Here's how the part is built. I have some questions about the finished solid (model axes, mm). A direction names the side the tool comes from. Coordinates: 2 decimals unless noted, no trailing zeros. Put each result on its own line as item: value.
```python
from build123d import *

# Parameters (mm, degrees)
SKETCH1_R           = 1.35
SKETCH1_R_2         = 1.3
BOSS_EXTRUDE1_DEPTH = 15.5
CUT_EXTRUDE1_DEPTH  = 6
FILLET1_R           = 3
CHAMFER1_SIZE       = 1.5
SKETCH3_W           = 7.93
SKETCH3_H           = 22
CUT_EXTRUDE2_DEPTH  = 8.3
SKETCH4_W           = 64.15
SKETCH4_H           = 2
CUT_EXTRUDE3_DEPTH  = 8.3


with BuildPart() as part:
    # Sketch1 → Boss-Extrude1 (new body)
    with BuildSketch(Plane.XY):
        with BuildLine():
            Line((-36.4, 19.96), (-36.4, 28))
            Line((-36.4, 28), (-39.5, 28))
            ThreePointArc((-39.5, 28), (-41.621320344, 27.121320344), (-42.5, 25))
            Line((-42.5, 25), (-42.5, -25))
            ThreePointArc((-42.5, -25), (-41.621320344, -27.121320344), (-39.5, -28))
            Line((-39.5, -28), (27.64, -28))
            Line((27.64, -28), (27.64, 8.8))
            Line((27.64, 8.8), (23.15, 8.8))
            Line((23.15, 8.8), (23.15, 28))
            Line((23.15, 28), (16.4, 28))
            Line((16.4, 28), (16.4, 21.51))
            Line((16.4, 21.51), (22.004438923, 21.51))
            Line((22.004438923, 21.51), (22.004438923, 15.51))
            Line((22.004438923, 15.51), (16.004438923, 15.51))
            Line((16.004438923, 15.51), (16.004438923, 19.96))
            Line((16.004438923, 19.96), (-36.4, 19.96))
        make_face()
        with Locations((-39, -24.5)):
            Circle(SKETCH1_R, mode=Mode.SUBTRACT)
        with Locations((19, -24.5)):
            Circle(SKETCH1_R, mode=Mode.SUBTRACT)
        with BuildLine():
            ThreePointArc((1.975, -8.92), (3.975, -6.92), (5.975, -8.92))
            Line((5.975, -8.92), (5.975, -24))
            ThreePointArc((5.975, -24), (3.975, -26), (1.975, -24))
            Line((1.975, -24), (1.975, -8.92))
        make_face(mode=Mode.SUBTRACT)
        with BuildLine():
            ThreePointArc((-40.535, 7.54), (-38.535, 9.54), (-36.535, 7.54))
            Line((-36.535, 7.54), (-36.535, -7.54))
            ThreePointArc((-36.535, -7.54), (-38.535, -9.54), (-40.535, -7.54))
            Line((-40.535, -7.54), (-40.535, 7.54))
        make_face(mode=Mode.SUBTRACT)
        with Locations((-39, 24.5)):
            Circle(SKETCH1_R_2, mode=Mode.SUBTRACT)
        with Locations((19, 24.5)):
            Circle(SKETCH1_R, mode=Mode.SUBTRACT)
        Polygon((22.004438923, 21.51), (16.4, 21.51), (16.4, 19.96), (16.004438923, 19.96), (16.004438923, 15.51), (22.004438923, 15.51), align=None)
    extrude(amount=BOSS_EXTRUDE1_DEPTH)

    # Sketch2 → Cut-Extrude1 (cut)
    with BuildSketch(Plane(origin=(0, 0, 0), x_dir=(-1, 0, 0), z_dir=(0, 0, -1))):
        Polygon((-16.4, 19.96), (-16.4, 21), (-23.15, 21), (-23.15, 8.8), (-27.64, 8.8), (-27.64, -28), (-22.5, -28), (-22.5, -21), (-15.5, -21), (-15.5, -28), (35.5, -28), (35.5, -21), (42.5, -21), (42.5, 21), (36.4, 21), (36.4, 19.96), align=None)
        with BuildLine():
            Line((-1.975, -8.92), (-1.975, -24))
            ThreePointArc((-1.975, -24), (-3.975, -26), (-5.975, -24))
            Line((-5.975, -24), (-5.975, -8.92))
            ThreePointArc((-5.975, -8.92), (-3.975, -6.92), (-1.975, -8.92))
        make_face(mode=Mode.SUBTRACT)
        with BuildLine():
            Line((40.535, 7.54), (40.535, -7.54))
            ThreePointArc((40.535, -7.54), (38.535, -9.54), (36.535, -7.54))
            Line((36.535, -7.54), (36.535, 7.54))
            ThreePointArc((36.535, 7.54), (38.535, 9.54), (40.535, 7.54))
        make_face(mode=Mode.SUBTRACT)
    extrude(amount=-CUT_EXTRUDE1_DEPTH, mode=Mode.SUBTRACT)

    # Fillet1
    fillet1_edges = [part.edges().sort_by_distance(p)[0] for p in [
        (-36.4, 19.96, 10.75),
        (16.4, 19.96, 10.75),
    ]]
    fillet(fillet1_edges, radius=FILLET1_R)

    # Chamfer1
    chamfer1_edges = [part.edges().sort_by_distance(p)[0] for p in [
        (-37.95, 28, 15.5),
        (-41.621320344, 27.121320344, 15.5),
        (-42.5, 0, 15.5),
        (-41.621320344, -27.121320344, 15.5),
        (-5.93, -28, 15.5),
        (19.775, 28, 15.5),
    ]]
    chamfer(chamfer1_edges, length=CHAMFER1_SIZE)

    # Sketch3 → Cut-Extrude2 (cut)
    with BuildSketch(Plane.XY.offset(15.5)):
        with Locations((-38.535, 0)):
            Rectangle(SKETCH3_W, SKETCH3_H)
    extrude(amount=-CUT_EXTRUDE2_DEPTH, mode=Mode.SUBTRACT)

    # Sketch4 → Cut-Extrude3 (cut)
    with BuildSketch(Plane.XY.offset(15.5)):
        with Locations((-8.925, 18.65)):
            Rectangle(SKETCH4_W, SKETCH4_H)
        with Locations((-8.925, 14.65)):
            Rectangle(SKETCH4_W, SKETCH4_H)
        with Locations((-8.925, 10.65)):
            Rectangle(SKETCH4_W, SKETCH4_H)
        with Locations((-8.925, 6.65)):
            Rectangle(SKETCH4_W, SKETCH4_H)
        with Locations((-8.925, 2.65)):
            Rectangle(SKETCH4_W, SKETCH4_H)
        with Locations((-8.925, -1.35)):
            Rectangle(SKETCH4_W, SKETCH4_H)
        with Locations((-8.925, -5.35)):
            Rectangle(SKETCH4_W, SKETCH4_H)
        with Locations((-8.925, -9.35)):
            Rectangle(SKETCH4_W, SKETCH4_H)
        with Locations((-8.925, -13.35)):
            Rectangle(SKETCH4_W, SKETCH4_H)
        with Locations((-8.925, -17.35)):
            Rectangle(SKETCH4_W, SKETCH4_H)
        with Locations((-8.925, -21.35)):
            Rectangle(SKETCH4_W, SKETCH4_H)
    extrude(amount=-CUT_EXTRUDE3_DEPTH, mode=Mode.SUBTRACT)


solid = part.part
```
Item 1: Please list where these lines run through material, in increasing order: line 1 along Y through (x, z) = (-39, 6.5); line 2 along X through (y, z) = (-17.5, 11.5); line 3 along X through (y, z) = (-23, 3.75). Write a range as from..to.
Output:
line 1: y = -28..-25.85, -23.15..-9.49, 9.49..23.2, 25.8..28
line 2: x = -42.5..-41, 23.15..27.64
line 3: x = -42.5..-35.5, 15.5..22.5
Item 2: For P1, Ø4, axis at x = -2.5, z = 5, coming from the -Y side; P2, Ø1.2, axis at x = -42, z = 12, coming from the -Y side; P3, Ø0.6, axis at x = 15, y = -13, coming from the +Z side; P4, Ø1.5, axis at x = 3.5, z = 13.5, coming from the +Y side, each with a flat end and sliding along its axis, tell me the tip position at first contact or that it passes through.
Output:
P1: stops at y = -28
P2: stops at y = -27.32
P3: stops at z = 7.2
P4: stops at y = 19.96
Item 3: If we mould it in two halves opening along X, with no side actions, what happens to faces 6 (the flat face through (23.15, -9, 11)), 7 (the flat face through (-41, 15, 11)), 8 (the flat face through (-36.4, 25, 8))? For each: released by +X, released by -X, zero draft, split by the parting line, or undercut.
Output:
face 6: released by -X
face 7: released by +X
face 8: undercut
Item 4: Which directions (+Z, -Z, +X, -X, +Y, -Y) give clear straight access to the entire face, cutting with the end or side of a thin tool? Please do faces 1 (the flat face through (-20, -17, 7.2)), 2 (the flat face through (25, 8.8, 11)), 3 (the flat face through (-35.5, -25, 3)), 4 (the flat face through (-6, 7.65, 11)), 5 (the cylindrical face through (3.93, -6.92, 10.68)).
Output:
face 1: +Z
face 2: +Z, -Z, +X, +Y
face 3: -Z, +Y, -Y
face 4: +Z, -X
face 5: +Z, -Z
Item 5: Imagine slicing it at A-A on x = 19. State how many separate pieces and enclosed holes the cut face has, then the cut area to 3 significant figures.
Output:
separate pieces: 3
enclosed holes: 0
area: 347 mm²
